from build123d import *

# Parameters (mm, degrees)
ESQUISSE1_R             = 9
ESQUISSE1_R_2           = 7.6
BOSS_EXTRU_1_DEPTH      = 5
ESQUISSE2_R             = 12.65
ESQUISSE2_R_2           = 7.6
BOSS_EXTRU_2_DEPTH      = 3
ESQUISSE3_R             = 11.65
ENL_V_MAT_EXTRU_1_DEPTH = 2
ESQUISSE4_R             = 1.5
ENL_V_MAT_EXTRU_2_DEPTH = 12


with BuildPart() as part:
    # Esquisse1 → Boss.-Extru.1 (new body)
    with BuildSketch(Plane(origin=(0, 0, 0), x_dir=(1, 0, 0), z_dir=(0, 1, 0))):
        with Locations(Location((0, 0, 0), (0, 0, 270))):
            Circle(ESQUISSE1_R)
        with Locations(Location((0, 0, 0), (0, 0, 270))):
            Circle(ESQUISSE1_R_2, mode=Mode.SUBTRACT)
    extrude(amount=BOSS_EXTRU_1_DEPTH)

    # Esquisse2 → Boss.-Extru.2 (add)
    with BuildSketch(Plane(origin=(0, 5, 0), x_dir=(1, 0, 0), z_dir=(0, 1, 0))):
        with Locations(Location((0, 0, 0), (0, 0, 270))):
            Circle(ESQUISSE2_R)
        with Locations(Location((0, 0, 0), (0, 0, 270))):
            Circle(ESQUISSE2_R_2, mode=Mode.SUBTRACT)
    extrude(amount=BOSS_EXTRU_2_DEPTH)

    # Esquisse3 → Enlèv. mat.-Extru.1 (cut)
    with BuildSketch(Plane(origin=(0, 8, 0), x_dir=(1, 0, 0), z_dir=(0, 1, 0))):
        with Locations(Location((0, 0, 0), (0, 0, 270))):
            Circle(ESQUISSE3_R)
    extrude(amount=-ENL_V_MAT_EXTRU_1_DEPTH, mode=Mode.SUBTRACT)

    # Esquisse4 → Enlèv. mat.-Extru.2 (cut)
    with BuildSketch(Plane.XY):
        with Locations(Location((0, 2.5, 0), (0, 0, 90))):
            Circle(ESQUISSE4_R)
    extrude(amount=-ENL_V_MAT_EXTRU_2_DEPTH, mode=Mode.SUBTRACT)


solid = part.part
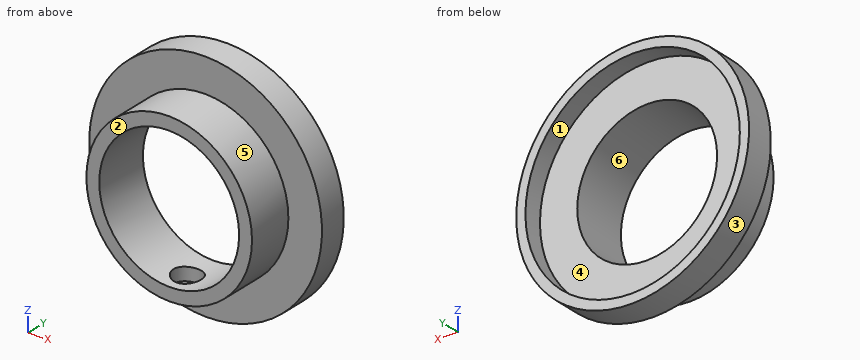
Work out the finished part from the listing and answer in its coordinate system (mm). Face numbers are marked on the shaded views. A direction names the side the tool comes from. Coordinates: 2 decimals unless noted, no trailing zeros. Loops run counter-clockwise (first coordinate to the right, second up) from the corner with the lowest first, then second, coordinate; pieces in that order, holes last. Notation, with made-up numbers: M -9,40 L 8,40 A26 ccw 8,75 Z; hole C 53,27 d10. An arc over 180 degrees is marked long. Answer in a Markdown table with one row per item. Add a question column.
1. Flat-ended cylindrical pins translate along their axes: P1, Ø3, axis at y = 1.5, z = 7.5, coming from the -X side; P2, Ø4, axis at y = 2.5, z = 5.5, coming from the +X side; P3, Ø7, axis at x = 5.5, z = 3.5, coming from the +Y side. Find the tip coordinate at first contact, or state that the pin passes through.
2. Find section C-C, the plane x = -7.25. Write down the section's boundary in (y, z), then the cut area to 3 significant figures.
3. Find section A-A, the plane z = 0. Write down the section's boundary in (x, y).
4. Find section D-D, the plane y = 0.5. Write down the section's boundary in (x, z).
5. Consider L1, parallel to X at y = 7.3, z = 0; L2, parallel to X at y = 1.5, z = 0; L3, parallel to Y at x = -11, z = -3. Determine where each line is inside the solid, lowest interval first.
6. Find section B-B, the plane x = 0. Write down the section's boundary in (y, z).
7. The mould has two halves that part along X. Classify the marked faces 1, 2 and 3: pulls with the +X half, pulls with the -X half, needs draft (parallel to the pull), parting line crosses it, or undercut.
8. A tool of negligible diameter and unlimited length cuts with its end or side. For the marked faces 4, 5 and 6, from which of +Z, -Z, +X, -X, +Y, -Y can it reach the whole face along a straight path? Write none if from no direction.
Reported:
| question | item | result |
|---|---|---|
| 1 | P1 | stops at x = -6.71 |
| 1 | P2 | stops at x = 8.29 |
| 1 | P3 | stops at y = 6 |
| 2 | outline | M 0,-5.33 L 5,-5.33 L 5,-10.37 L 8,-10.37 L 8,-9.12 L 6,-9.12 L 6,-2.28 L 0,-2.28 Z; M 0,2.28 L 6,2.28 L 6,9.12 L 8,9.12 L 8,10.37 L 5,10.37 L 5,5.33 L 0,5.33 Z |
| 2 | area | 51.7 mm^2 |
| 3 | outline | M -12.65,5 L -9,5 L -9,0 L -7.6,0 L -7.6,6 L -11.65,6 L -11.65,8 L -12.65,8 Z; M 7.6,0 L 9,0 L 9,5 L 12.65,5 L 12.65,8 L 11.65,8 L 11.65,6 L 7.6,6 Z |
| 4 | outline | C 0,0 d18; hole C 0,0 d15.2 |
| 5 | L1 | x = -12.65 to -11.65, 11.65 to 12.65 |
| 5 | L2 | x = -9 to -7.6, 7.6 to 9 |
| 5 | L3 | y = 5 to 6 |
| 6 | outline | M 0,-9 L 1,-9 L 1,-7.6 L 0,-7.6 Z; M 0,7.6 L 6,7.6 L 6,11.65 L 8,11.65 L 8,12.65 L 5,12.65 L 5,9 L 0,9 Z; M 4,-9 L 5,-9 L 5,-12.65 L 8,-12.65 L 8,-11.65 L 6,-11.65 L 6,-7.6 L 4,-7.6 Z |
| 7 | face 1 | undercut |
| 7 | face 2 | needs draft |
| 7 | face 3 | parting line crosses it |
| 8 | face 4 | +Y |
| 8 | face 5 | -Y |
| 8 | face 6 | +Y, -Y |
